Geometry check sheet. Reference: the model listing, model coordinates, mm. A direction names the side the tool comes from. Give positions to 0.01 mm unless a question says otherwise; leave off trailing zeros. Order: outer loops, then holes, each group sorted by start corner. A loop starts at its lowest first (then second) coordinate and runs counter-clockwise, first axis right, second up. Notation, with made-up numbers: M 24,-38 L 32,-38 A12 cw 32,-25 Z; hole C 24.5,88 d10. An arc over 180 degrees is marked long. Answer as a JSON object with one key per item and string values. Group by question number.
from build123d import *

# Parameters (mm, degrees)
EXTRUSION1_DEPTH             = 10
ENL_V_MAT_EXTRU_1_DEPTH      = 300
R_P_TITION_CIRCULAIRE1_COUNT = 4


with BuildPart() as part:
    # Esquisse1 → Extrusion1 (new body, symmetric)
    with BuildSketch(Plane.XY):
        with BuildLine():
            Line((-6, 5), (-6, -5))
            ThreePointArc((-6, -5), (-5.707106781, -5.707106781), (-5, -6))
            Line((-5, -6), (5, -6))
            ThreePointArc((5, -6), (5.707106781, -5.707106781), (6, -5))
            Line((6, -5), (6, 5))
            ThreePointArc((6, 5), (5.707106781, 5.707106781), (5, 6))
            Line((5, 6), (-5, 6))
            ThreePointArc((-5, 6), (-5.707106781, 5.707106781), (-6, 5))
        make_face()
    extrude(amount=EXTRUSION1_DEPTH, both=True)

    # Esquisse3 → Enl_v. mat.-Extru.1 (cut)
    with BuildSketch(Plane.XY.offset(10)):
        Polygon((6, 2), (4.8, 2), (4.8, 4), (2, 1), (2, -1), (4.8, -4), (4.8, -2), (6, -2), align=None)
    enl_v_mat_extru_1 = extrude(amount=-ENL_V_MAT_EXTRU_1_DEPTH, mode=Mode.SUBTRACT)

    # R_p_tition circulaire1: Enl_v. mat.-Extru.1 ×4 about axis
    r_p_tition_circulaire1_axis = Axis((0, 0, 0), (0, 0, 1))
    for i in range(1, R_P_TITION_CIRCULAIRE1_COUNT):
        add(enl_v_mat_extru_1.rotate(r_p_tition_circulaire1_axis, i * 360 / R_P_TITION_CIRCULAIRE1_COUNT), mode=Mode.SUBTRACT)


solid = part.part
1. Cross-section at B-B (x = 5.25). Record the cut outline in (y, z), and give its area (3 significant figures).
2. Cross-section at A-A (y = 2.5). Record the cut outline in (x, z), and give its area (3 significant figures).
3. Access from +Z, -Z, +X, -X, +Y, -Y to the whole of each face (thin tool, end or side, straight path). Record for faces 4 (the flat face through (5, 2, 0)), 5 (the flat face through (0, 2, 0)), 6 (the flat face through (-5, 2, 0)), 7 (the flat face through (4.8, 3, 0)).
4. Release check for a two-part mould opening along X. For faces 1 (the flat face through (5, -2, 0)), 2 (the cylindrical face through (-5.699, 5.715, 0.14)), 3 (the flat face through (-2.5, -3.4, 0.1)) record: released by +X, released by -X, zero draft, split by the parting line, or undercut.
5. Depth check by flat-ended pin: pin 1 (0.6 mm diameter, centred on x = 5.5, z = 5, fed in from -Y); pin 2 (1 mm diameter, centred on x = 0, z = 2, fed in from +Y); pin 3 (2 mm diameter, centred on y = -0.5, z = -4, fed in from +X). Enter the tip coordinate at first touch or a pass-through.
6. Cross-section at D-D (x = 0). Record the cut outline in (y, z).
7. Thickness scan on line 1 along X through (y, z) = (-3.75, 6) (3 decimals); line 2 along Y through (x, z) = (-5, 1.75). Record the ranges inside material, lowest first. Write a range as [from, to].
Report:
{
 "1": {"outline": "M -5.97,-10 L -2,-10 L -2,10 L -5.97,10 Z; M 2,-10 L 5.97,-10 L 5.97,10 L 2,10 Z", "area": "159 mm2"},
 "2": {"outline": "M -6,-10 L -4.8,-10 L -4.8,10 L -6,10 Z; M -3.4,-10 L -1.54,-10 L -1.54,10 L -3.4,10 Z; M 1.54,-10 L 3.4,-10 L 3.4,10 L 1.54,10 Z; M 4.8,-10 L 6,-10 L 6,10 L 4.8,10 Z", "area": "123 mm2"},
 "3": {"face 4": "+Z, -Z, +X", "face 5": "+Z, -Z, +Y", "face 6": "+Z, -Z, -X", "face 7": "+Z, -Z"},
 "4": {"face 1": "zero draft", "face 2": "released by -X", "face 3": "undercut"},
 "5": {"pin 1": "stops at y = -5.98", "pin 2": "stops at y = 2", "pin 3": "stops at x = 2.47"},
 "6": {"outline": "M -2,-10 L 2,-10 L 2,10 L -2,10 Z"},
 "7": {"line 1": "x = [-6, -4.8], [-4.567, -2.875], [2.875, 4.567], [4.8, 6]", "line 2": "y = [-6, -2], [2, 6]"}
}
